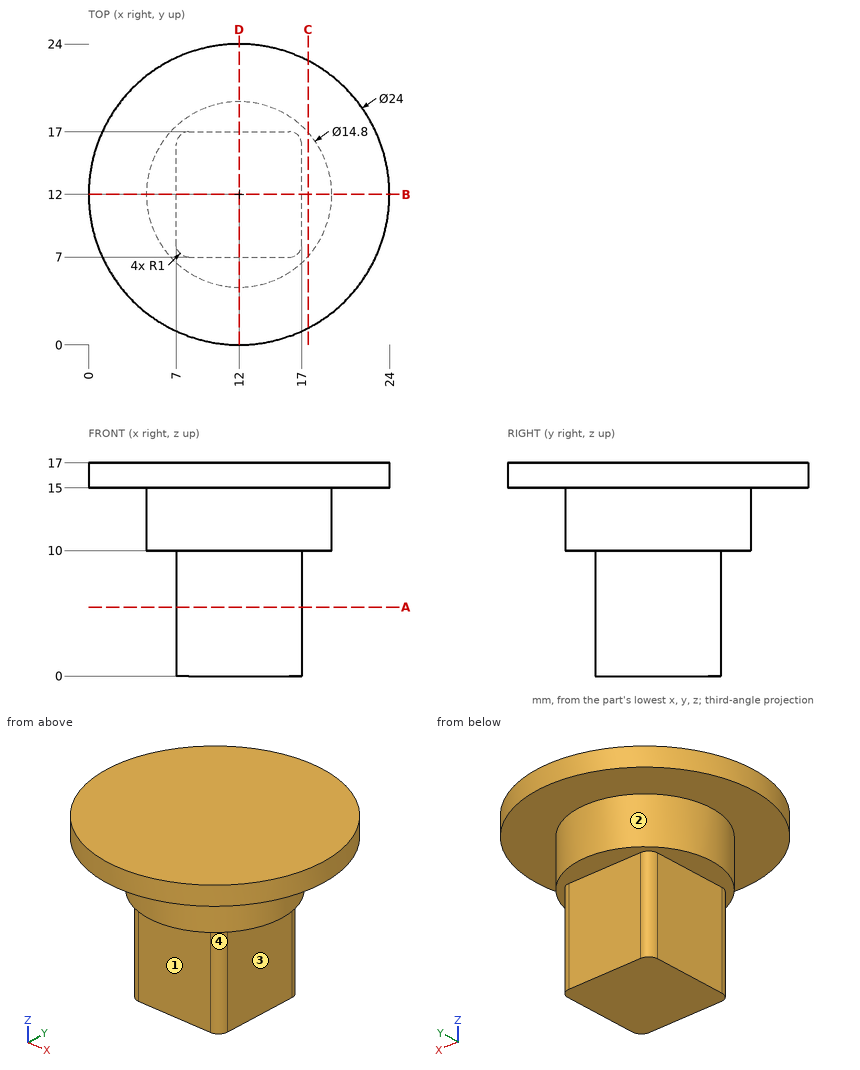
Job drawing, mm, ordinate dimensions from the low corner. One solid piece. A direction names the side the tool comes from. Round coordinates to 2 decimals unless told otherwise and drop trailing zeros. Loops run counter-clockwise (first coordinate to the right, second up) from the corner with the lowest first, then second, coordinate; pieces in that order, holes last.
Item 1: 3-axis set-ups, long thin cutter, end or side, ignore diameter. For the marked faces 1, 2, 3 and 4: which of +Z, -Z, +X, -X, +Y, -Y reach the whole face in a straight line?
Item 2: Cut at C-C, the plane x = 17.5. Give the cut face in (y, z), then the cut area to 3 significant figures.
Item 3: Drop flat-ended pins along their axis: P1, Ø6, axis at x = 7.5, z = 8.5, coming from the -Y side; P2, Ø9, axis at y = 12, z = 4.5, coming from the -X side; P3, Ø2.5, axis at x = 10.5, z = 4, coming from the +Y side; P4, Ø12, axis at x = 6, y = 13.5, coming from the -Z side. Give the stop position or say it passes through.
Item 4: Drill centre lines: line 1 (X direction, y = 11.5, z = 4.75); line 2 (Z direction, x = 16, y = 22); line 3 (Z direction, x = 14, y = 19). Where is each one in solid material? Low to high.
Item 5: Cut at A-A, the plane z = 5.5. Give the cut face in (x, y), then the cut area to 3 significant figures.
Item 6: Cut at B-B, the plane y = 12. Give the cut face in (x, z).
A:
1. face 1: -Z, +X, -X, -Y
1. face 2: -Z
1. face 3: -Z, +X, +Y, -Y
1. face 4: -Z, +X, -Y
2. outline: (1.33, 15) - (7.05, 15) - (7.05, 10) - (16.95, 10) - (16.95, 15) - (22.67, 15) - (22.67, 17) - (1.33, 17) - close
2. area: 92.2 mm2
3. P1: stops at y = 4.85
3. P2: stops at x = 7
3. P3: stops at y = 17
3. P4: stops at z = 0
4. line 1: x = 7 to 17
4. line 2: z = 15 to 17
4. line 3: z = 10 to 17
5. outline: (7, 8) arc R1 ccw to (8, 7) - (16, 7) arc R1 ccw to (17, 8) - (17, 16) arc R1 ccw to (16, 17) - (8, 17) arc R1 ccw to (7, 16) - close
5. area: 99.1 mm2
6. outline: (0, 15) - (4.6, 15) - (4.6, 10) - (7, 10) - (7, 0) - (17, 0) - (17, 10) - (19.4, 10) - (19.4, 15) - (24, 15) - (24, 17) - (0, 17) - close
